Read the model definition and answer for the solid it produces. Units are mm, in the model's axes. A direction names the side the tool comes from. Coordinates: 2 decimals unless noted, no trailing zeros.
(1) The part is cut by section A-A, the plane y = 0.9. State how many separate pieces and enclosed holes the cut face has, and give its area (3 significant figures).
(2) Which of the six approach directions +Z, -Z, +X, -X, +Y, -Y give full straight-line access (tool end or side, diameter ignored) to faces 1 (the cylindrical face through (-61.357, 2.028, -18.407)), 2 (the flat face through (23.5, 2.5, -36.1)), 3 (the flat face through (-91.406, 2, 9))?
(3) Straight lines are drawn through the part: line 1 along X through (y, z) = (1.5, 53); line 2 along X through (y, z) = (2.1, -12). For each, find the intervals that lie inside material, in ascending order.
(4) Given pin 1 (1.4 mm diameter, centred on x = 27, z = 53.5, fed in from +Y), flat-ended and moving along its own axis, determine where the tip first touches the part or whether it passes through.
```python
from build123d import *

# Parameters (mm, degrees)
SKETCH1_W           = 122
SKETCH1_H           = 97.5
BOSS_EXTRUDE1_DEPTH = 4
SKETCH2_R           = 1.4
CUT_EXTRUDE1_DEPTH  = 4
SKETCH3_R           = 2.4
CUT_EXTRUDE2_DEPTH  = 1.5
CUT_EXTRUDE3_DEPTH  = 4


with BuildPart() as part:
    # Sketch1 → Boss-Extrude1 (new body)
    with BuildSketch(Plane(origin=(0, 0, 0), x_dir=(1, 0, 0), z_dir=(0, 1, 0))):
        with Locations((-30.40625, -8.671875)):
            Rectangle(SKETCH1_W, SKETCH1_H)
    extrude(amount=BOSS_EXTRUDE1_DEPTH)

    # Sketch2 → Cut-Extrude1 (cut)
    with BuildSketch(Plane(origin=(0, 4, 0), x_dir=(1, 0, 0), z_dir=(0, 1, 0))):
        with Locations(Location((-86.90625, -53.261875, 0), (0, 0, 270))):
            Circle(SKETCH2_R)
        with Locations(Location((-86.90625, 14.538125, 0), (0, 0, 270))):
            Circle(SKETCH2_R)
        with Locations(Location((26.09375, 14.538125, 0), (0, 0, 270))):
            Circle(SKETCH2_R)
        with Locations(Location((26.09375, -53.261875, 0), (0, 0, 270))):
            Circle(SKETCH2_R)
        with Locations(Location((-85.90625, 36.078125, 0), (0, 0, 270))):
            Circle(SKETCH2_R)
        with Locations(Location((25.09375, 36.078125, 0), (0, 0, 270))):
            Circle(SKETCH2_R)
    extrude(amount=-CUT_EXTRUDE1_DEPTH, mode=Mode.SUBTRACT)

    # Sketch3 → Cut-Extrude2 (cut)
    with BuildSketch(Plane(origin=(0, 4, 0), x_dir=(1, 0, 0), z_dir=(0, 1, 0))):
        with Locations(Location((-86.90625, 14.538125, 0), (0, 0, 270))):
            Circle(SKETCH3_R)
        with Locations(Location((-86.90625, -53.261875, 0), (0, 0, 270))):
            Circle(SKETCH3_R)
        with Locations(Location((26.09375, -53.261875, 0), (0, 0, 270))):
            Circle(SKETCH3_R)
        with Locations(Location((26.09375, 14.538125, 0), (0, 0, 270))):
            Circle(SKETCH3_R)
        with Locations(Location((-85.90625, 36.078125, 0), (0, 0, 270))):
            Circle(SKETCH3_R)
        with Locations(Location((25.09375, 36.078125, 0), (0, 0, 270))):
            Circle(SKETCH3_R)
    extrude(amount=-CUT_EXTRUDE2_DEPTH, mode=Mode.SUBTRACT)

    # Sketch4 → Cut-Extrude3 (cut)
    with BuildSketch(Plane(origin=(0, 4, 0), x_dir=(1, 0, 0), z_dir=(0, 1, 0))):
        with BuildLine():
            Line((-1.65625, 16.157315761), (-1.65625, 12.586287383))
            ThreePointArc((-1.65625, 12.586287383), (0.59375, 4.18990801), (2.84375, 12.586287383))
            Line((2.84375, 12.586287383), (2.84375, 16.157315761))
            ThreePointArc((2.84375, 16.157315761), (0.59375, 18.407315761), (-1.65625, 16.157315761))
        make_face()
        with BuildLine():
            Line((-63.65625, 16.157315761), (-63.65625, 12.586287383))
            ThreePointArc((-63.65625, 12.586287383), (-61.40625, 4.18990801), (-59.15625, 12.586287383))
            Line((-59.15625, 12.586287383), (-59.15625, 16.157315761))
            ThreePointArc((-59.15625, 16.157315761), (-61.40625, 18.407315761), (-63.65625, 16.157315761))
        make_face()
    extrude(amount=-CUT_EXTRUDE3_DEPTH, mode=Mode.SUBTRACT)


solid = part.part
```
Computed:
1. separate pieces: 1
1. enclosed holes: 8
1. area: 11,700 mm2
2. face 1: +Y, -Y
2. face 2: +Y
2. face 3: +Z, -Z, -X, +Y, -Y
3. line 1: x = -91.41 to -88.28, -85.53 to 24.72, 27.47 to 30.59
3. line 2: x = -91.41 to -64.45, -58.36 to -2.45, 3.64 to 30.59
4. pin 1: stops at y = 2.5
